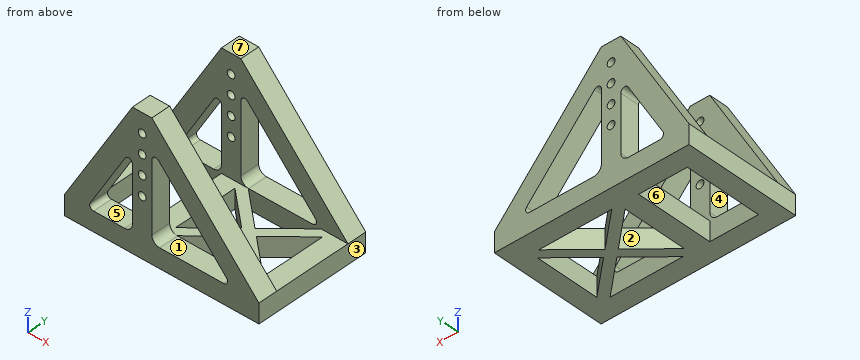
from build123d import *

# Parameters (mm, degrees)
F0_R        = 2.2479
F1_DEPTH    = 76.2
F2_W        = 50.8
F2_H        = 76.2
F3_DEPTH    = 254
F5_DEPTH    = 25.4
F6_T1_DEPTH = 12.7
F6_T3_DEPTH = 12.7
F7_T1_DEPTH = 12.7
F7_T3_DEPTH = 12.7
F8_R        = 2.54
F9_R        = 2.54
F10_DEPTH   = 254


# Not quite as in the source:
# - a fillet or chamfer that OpenCascade refuses, or shapes differently, is made with other operations: its cross-section is extruded or revolved along the edge and cut away or added


with BuildPart() as f1:
    # F0 (on Front) → F1 (new body)
    with BuildSketch(Plane.XZ):
        Polygon((-50.8, 0), (0, 0), (76.2, 0), (76.2, 12.7), (6.35, 88.9), (-6.35, 88.9), (-50.8, 12.7), align=None)
        Polygon((-6.35, 12.7), (-36.0971634445, 12.7), (-6.35, 63.6951373334), align=None, mode=Mode.SUBTRACT)
        with Locations((0, 38.1)):
            Circle(F0_R, mode=Mode.SUBTRACT)
        Polygon((6.35, 12.7), (6.35, 70.1053616754), (58.9715815358, 12.7), align=None, mode=Mode.SUBTRACT)
        with Locations((0, 50.8)):
            Circle(F0_R, mode=Mode.SUBTRACT)
        with Locations((0, 63.5)):
            Circle(F0_R, mode=Mode.SUBTRACT)
        with Locations((0, 76.2)):
            Circle(F0_R, mode=Mode.SUBTRACT)
    extrude(amount=F1_DEPTH)

    # F2 (on face) → F3 (cut)
    with BuildSketch(Plane(origin=(-50.8, 0, 0), x_dir=(0, -1, 0), z_dir=(-1, 0, 0))):
        with Locations((38.1, 50.8)):
            Rectangle(F2_W, F2_H)
    extrude(amount=-F3_DEPTH, mode=Mode.SUBTRACT)

    # F4 (on face) → F5 (cut)
    with BuildSketch(Plane.XY.offset(12.7)):
        Polygon((58.7209921515, -12.7), (11.1290078485, -12.7), (34.925, -33.8519930236), align=None)
        Polygon((34.925, -42.3480069764), (11.1290078485, -63.5), (58.7209921515, -63.5), align=None)
        Polygon((-36.0971634445, -12.7), (-38.1, -12.7), (-38.1, -63.5), (-36.0971634445, -63.5), (-6.35, -63.5), (-6.35, -12.7), align=None)
        Polygon((30.1459921515, -38.1), (6.35, -16.9480069764), (6.35, -59.2519930236), align=None)
        Polygon((63.5, -59.2519930236), (63.5, -16.9480069764), (39.7040078485, -38.1), align=None)
    extrude(amount=-F5_DEPTH, mode=Mode.SUBTRACT)

    # F6: fillet of radius 5.08 on 4 edges, made by hand

    # F6_s2 → F6_t1 (join)
    with BuildSketch(Plane.XZ.offset(63.5)):
        with BuildLine():
            ThreePointArc((-11.43, 12.7), (-7.8378975516, 14.1878975516), (-6.35, 17.78))
            Line((-6.35, 17.78), (-6.35, 12.7))
            Line((-6.35, 12.7), (-11.43, 12.7))
        make_face()
        with BuildLine():
            ThreePointArc((11.43, 12.7), (7.8378975516, 14.1878975516), (6.35, 17.78))
            Line((6.35, 17.78), (6.35, 12.7))
            Line((6.35, 12.7), (11.43, 12.7))
        make_face()
    extrude(amount=F6_T1_DEPTH)

    # F6_s4 → F6_t3 (join)
    with BuildSketch(Plane.XZ):
        with BuildLine():
            ThreePointArc((-11.43, 12.7), (-7.8378975516, 14.1878975516), (-6.35, 17.78))
            Line((-6.35, 17.78), (-6.35, 12.7))
            Line((-6.35, 12.7), (-11.43, 12.7))
        make_face()
        with BuildLine():
            ThreePointArc((11.43, 12.7), (7.8378975516, 14.1878975516), (6.35, 17.78))
            Line((6.35, 17.78), (6.35, 12.7))
            Line((6.35, 12.7), (11.43, 12.7))
        make_face()
    extrude(amount=F6_T3_DEPTH)

    # F7: fillet of radius 2.54 on 7 edges, made by hand

    # F7_s2 → F7_t1 (join)
    with BuildSketch(Plane.XZ.offset(63.5)):
        with BuildLine():
            ThreePointArc((-6.35, 54.2998790858), (-8.2271108528, 56.751853388), (-11.0839984083, 55.5797114907))
            Line((-11.0839984083, 55.5797114907), (-6.35, 63.6951373334))
            Line((-6.35, 63.6951373334), (-6.35, 54.2998790858))
        make_face()
        with BuildLine():
            ThreePointArc((55.0699360257, 16.9563405564), (55.5225489196, 14.2172353676), (53.1975645096, 12.7))
            Line((53.1975645096, 12.7), (58.9715815358, 12.7))
            Line((58.9715815358, 12.7), (55.0699360257, 16.9563405564))
        make_face()
        with BuildLine():
            ThreePointArc((10.7623715161, 65.291865476), (7.9691915647, 65.9427409692), (6.35, 63.5755249196))
            Line((6.35, 63.5755249196), (6.35, 70.1053616754))
            Line((6.35, 70.1053616754), (10.7623715161, 65.291865476))
        make_face()
    extrude(amount=F7_T1_DEPTH)

    # F7_s4 → F7_t3 (join)
    with BuildSketch(Plane.XZ):
        with BuildLine():
            ThreePointArc((6.35, 63.5755249196), (7.9691915647, 65.9427409692), (10.7623715161, 65.291865476))
            Line((10.7623715161, 65.291865476), (6.35, 70.1053616754))
            Line((6.35, 70.1053616754), (6.35, 63.5755249196))
        make_face()
        with BuildLine():
            ThreePointArc((-11.0839984083, 55.5797114907), (-8.2271108528, 56.751853388), (-6.35, 54.2998790858))
            Line((-6.35, 54.2998790858), (-6.35, 63.6951373334))
            Line((-6.35, 63.6951373334), (-11.0839984083, 55.5797114907))
        make_face()
        with BuildLine():
            ThreePointArc((55.0699360257, 16.9563405564), (55.5225489196, 14.2172353676), (53.1975645096, 12.7))
            Line((53.1975645096, 12.7), (58.9715815358, 12.7))
            Line((58.9715815358, 12.7), (55.0699360257, 16.9563405564))
        make_face()
        with BuildLine():
            ThreePointArc((-33.868927875, 16.5198324048), (-33.8774705343, 13.9749257548), (-31.6749294667, 12.7))
            Line((-31.6749294667, 12.7), (-36.0971634445, 12.7))
            Line((-36.0971634445, 12.7), (-33.868927875, 16.5198324048))
        make_face()
    extrude(amount=F7_T3_DEPTH)

    # F8
    f8_edges = [f1.edges().sort_by_distance(p)[0] for p in [
        (-36.097163, -69.85, 12.7),
    ]]
    fillet(f8_edges, radius=F8_R)

    # F9 (on face) → F10 (cut)
    with BuildSketch(Plane.XZ.offset(76.2)):
        with Locations((0, 76.2)):
            Circle(F9_R)
        with Locations((0, 63.5)):
            Circle(F9_R)
        with Locations((0, 50.8)):
            Circle(F9_R)
        with Locations((0, 38.1)):
            Circle(F9_R)
    extrude(amount=-F10_DEPTH, mode=Mode.SUBTRACT)


solid = f1.part
Check sheet for the modelled part. Datum: model origin and axes. Units: mm. Face numbers are marked on the shaded views. A direction names the side the tool comes from. Give positions to 0.01 mm unless a question says otherwise; leave off trailing zeros. Order: outer loops, then holes, each group sorted by start corner. A loop starts at its lowest first (then second) coordinate and runs counter-clockwise, first axis right, second up. Notation, with made-up numbers: (88.5, 88) - (138.5, 88) arc R19 ccw to (138.5, 102) - close; hole circle Ø9 at (44.5, 59). An arc over 180 degrees is marked (long way). Answer as CSV lines item,"result".
1. Go/stop test with flat-tipped pins: P1, Ø6, axis at x = -2, z = 31, coming from the +Y side; P2, Ø8, axis at y = -63, z = 76.5, coming from the +X side; P3, Ø10, axis at x = -21.5, y = -67, coming from the +Z side; P4, Ø6.5, axis at x = -21.5, y = -6.5, coming from the +Z side. Record where each tip stops, or that it passes through.
Result sheet:
P1,"y = 0"
P2,"x = 21.35"
P3,"z = 71.5"
P4,"z = 68.5"
2. Section check B-B (x = -25). Record the boundary of the cut face in (y, z).
Result sheet:
outline,"(-76.2, 0) - (-63.5, 0) - (-63.5, 12.7) - (-76.2, 12.7) - close; (-76.2, 31.72) - (-63.5, 31.72) - (-63.5, 56.93) - (-76.2, 56.93) - close; (-12.7, 0) - (0, 0) - (0, 12.7) - (-12.7, 12.7) - close; (-12.7, 31.72) - (0, 31.72) - (0, 56.93) - (-12.7, 56.93) - close"
3. Tool access check on the marked faces 1, 2 and 3. Record the directions out of +Z, -Z, +X, -X, +Y, -Y that give a thin tool (end or side, any length) a straight path to the whole face; none if there is none.
Result sheet:
face 1,"+Y, -Y"
face 2,"+Z, -Z"
face 3,"+Z, -Z, +X, +Y, -Y"
4. Section check A-A (z = 76.2). Record the boundary of the cut face in (x, y).
Result sheet:
outline,"(-13.76, -76.2) - (-2.54, -76.2) - (-2.54, -63.5) - (-13.76, -63.5) - close; (-13.76, -12.7) - (-2.54, -12.7) - (-2.54, 0) - (-13.76, 0) - close; (2.54, -76.2) - (17.99, -76.2) - (17.99, -63.5) - (2.54, -63.5) - close; (2.54, -12.7) - (17.99, -12.7) - (17.99, 0) - (2.54, 0) - close"
5. Section check C-C (y = -28). Record the boundary of the cut face in (x, z).
Result sheet:
outline,"(-50.8, 0) - (-38.1, 0) - (-38.1, 12.7) - (-50.8, 12.7) - close; (-6.35, 0) - (6.35, 0) - (6.35, 12.7) - (-6.35, 12.7) - close; (18.78, 0) - (28.34, 0) - (28.34, 12.7) - (18.78, 12.7) - close; (41.51, 0) - (51.07, 0) - (51.07, 12.7) - (41.51, 12.7) - close; (63.5, 0) - (76.2, 0) - (76.2, 12.7) - (63.5, 12.7) - close"
6. Scan lines: probe 1 along Z at (x, y) = (0, -68.75); probe 2 along Y at (x, z) = (31, 46.5); probe 3 along X at (y, z) = (-69, 22) (3 decimals). Record each from-to range of solid material in increasing order. Write a range as from..to.
Result sheet:
probe 1,"0..35.56, 40.64..48.26, 53.34..60.96, 66.04..73.66, 78.74..88.9"
probe 2,"-76.2..-63.5, -12.7..0"
probe 3,"-45.375..-30.672, -6.35..6.35, 50.447..67.675"
7. Section check D-D (z = 46). Record the boundary of the cut face in (x, y) (3 decimals), then the cut area to 3 significant figures.
Result sheet:
outline,"(-31.375, -76.2) - (-16.672, -76.2) - (-16.672, -63.5) - (-31.375, -63.5) - close; (-31.375, -12.7) - (-16.672, -12.7) - (-16.672, 0) - (-31.375, 0) - close; (-6.35, -76.2) - (6.35, -76.2) - (6.35, -63.5) - (-6.35, -63.5) - close; (-6.35, -12.7) - (6.35, -12.7) - (6.35, 0) - (-6.35, 0) - close; (28.447, -76.2) - (45.675, -76.2) - (45.675, -63.5) - (28.447, -63.5) - close; (28.447, -12.7) - (45.675, -12.7) - (45.675, 0) - (28.447, 0) - close"
area,"1,130 mm²"
8. Mould release check, pull along Z, two halves, no side actions. Record for the marked faces 4, 5, 6 and 7: released by +Z, released by -Z, zero draft, split by the parting line, or undercut.
Result sheet:
face 4,"undercut"
face 5,"undercut"
face 6,"zero draft"
face 7,"released by +Z"
